Here's the drawing with two shaded views (mm, measured from the low corner). I have some questions. Round coordinates to 2 decimals unless told otherwise and drop trailing zeros. Order: outer loops, then holes, each group sorted by start corner. A loop starts at its lowest first (then second) coordinate and runs counter-clockwise, first axis right, second up. Notation, with made-up numbers: (8.25, 6) -> (15.25, 6) arc R12 cw to (15.25, 21) -> close; hole circle Ø9 at (-4, 49.5). An arc over 180 degrees is marked (long way). Use a Markdown table: item, result. Add a question column.
Q1. If we section it at B-B on x = 115.5: List the corners of the cut face in (y, z) for me (1 decimal).
Q2. If we section it at A-A on z = 4.3: Give the number of separate pieces and of enclosed holes in the cut face.
Q3. If we section it at C-C on y = 6: List the corners of the cut face in (x, z) for me (1 decimal), plus the area to 3 significant figures.
Q4. I need wall thicknesses on line 1 along X through (y, z) = (13.25, 5.4) (1 decimal); line 2 along X through (y, z) = (11.5, 0.6); line 3 along Y through (x, z) = (210.5, 4.85). Which ranges of each line are inside material? Lowest first, please. Write a range as [from, to].
Q5. I'm going to push flat-ended pins straight in: pin 1 Ø1.5 at (y, z) = (2, 4) entering from +X; pin 2 Ø2.5 at (y, z) = (24, 2.5) entering from -X; pin 3 Ø1.7 at (x, z) = (23, 3) entering from +Y; pin 4 Ø2.5 at (x, y) = (123.82, 12.48) entering from +Z. Where does each tip first touch, or does it pass through?
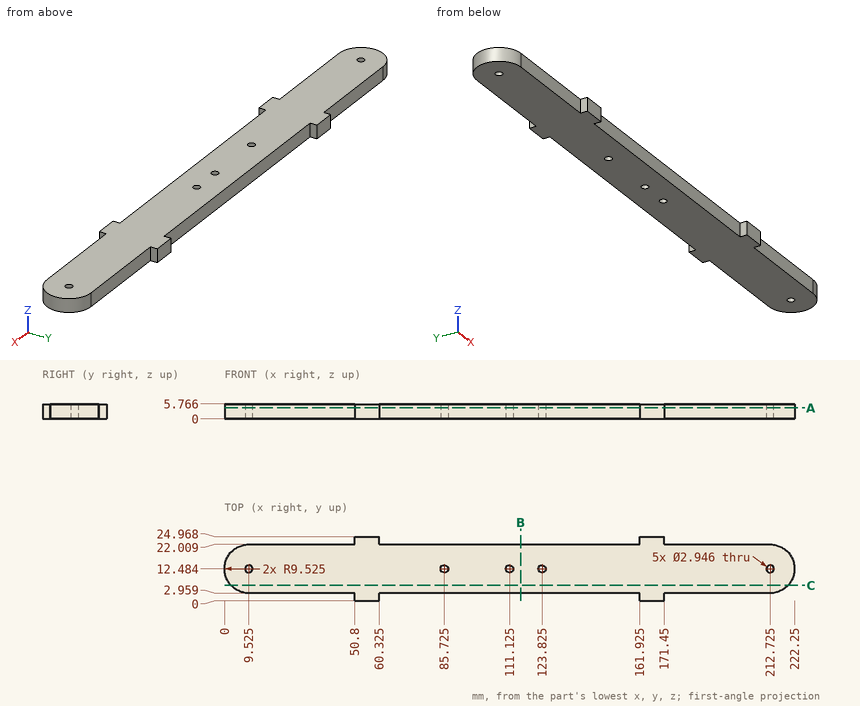
Answer below:
| question | item | result |
|---|---|---|
| 1 | outline | (3, 0) -> (22, 0) -> (22, 5.8) -> (3, 5.8) -> close |
| 2 | separate pieces | 1 |
| 2 | enclosed holes | 5 |
| 3 | outline | (2.5, 0) -> (219.7, 0) -> (219.7, 5.8) -> (2.5, 5.8) -> close |
| 3 | area | 1,250 mm² |
| 4 | line 1 | [0, 8.3], [10.8, 84.5], [87, 109.9], [112.4, 122.6], [125.1, 211.5], [214, 222.2] |
| 4 | line 2 | [0.05, 8.43], [10.62, 84.63], [86.82, 110.03], [112.22, 122.73], [124.92, 211.63], [213.82, 222.2] |
| 4 | line 3 | [2.96, 22.01] |
| 5 | pin 1 | x = 171.45 |
| 5 | pin 2 | x = 50.8 |
| 5 | pin 3 | y = 22.01 |
| 5 | pin 4 | through |
